```python
from build123d import *

# Parameters (mm, degrees)
DODANIE_WYCI_GNI_CIE1_DEPTH = 10
SZKIC2_R                    = 1.75
WYTNIJ_WYCI_GNI_CIE1_DEPTH  = 10


with BuildPart() as part:
    # Szkic1 → Dodanie-wyciągnięcie1 (new body)
    with BuildSketch(Plane(origin=(0, 0, 0), x_dir=(1, 0, 0), z_dir=(0, 1, 0))):
        with BuildLine():
            Line((22, -25), (-22, -25))
            ThreePointArc((-22, -25), (-24.121320344, -24.121320344), (-25, -22))
            Line((-25, -22), (-25, 22))
            ThreePointArc((-25, 22), (-24.121320344, 24.121320344), (-22, 25))
            Line((-22, 25), (22, 25))
            ThreePointArc((22, 25), (24.121320344, 24.121320344), (25, 22))
            Line((25, 22), (25, -22))
            ThreePointArc((25, -22), (24.121320344, -24.121320344), (22, -25))
        make_face()
    extrude(amount=DODANIE_WYCI_GNI_CIE1_DEPTH)

    # Szkic2 → Wytnij-wyciągnięcie1 (cut)
    with BuildSketch(Plane(origin=(0, 10, 0), x_dir=(1, 0, 0), z_dir=(0, 1, 0))):
        with Locations(Location((-20, 20, 0), (0, 0, 270))):
            Circle(SZKIC2_R)
        with Locations(Location((20, 20, 0), (0, 0, 270))):
            Circle(SZKIC2_R)
        with Locations(Location((20, -20, 0), (0, 0, 270))):
            Circle(SZKIC2_R)
        with Locations(Location((-20, -20, 0), (0, 0, 270))):
            Circle(SZKIC2_R)
        with BuildLine():
            Line((19.949804326, -0.416088747), (8.887895851, -0.416088747))
            ThreePointArc((8.887895851, -0.416088747), (8.238797705, -0.655384076), (7.900351868, -1.258745553))
            ThreePointArc((7.900351868, -1.258745553), (4.101739563, -6.868459256), (-2.638482905, -7.552377636))
            ThreePointArc((-2.638482905, -7.552377636), (-3.348489276, -7.571518902), (-3.866696101, -8.057252494))
            Line((-3.866696101, -8.057252494), (-8.71289149, -17.970981564))
            ThreePointArc((-8.71289149, -17.970981564), (-8.751315605, -18.759947091), (-8.20521309, -19.330661607))
            ThreePointArc((-8.20521309, -19.330661607), (10.963128103, -17.911164736), (20.947294543, -1.486893185))
            ThreePointArc((20.947294543, -1.486893185), (20.681516168, -0.734474647), (19.949804326, -0.416088747))
        make_face()
        with BuildLine():
            Line((19.918829975, 1.449846448), (8.910113622, 0.686816973))
            ThreePointArc((8.910113622, 0.686816973), (8.230490402, 0.892390127), (7.858638328, 1.497265385))
            ThreePointArc((7.858638328, 1.497265385), (3.997324324, 6.929747344), (-2.638482905, 7.552377636))
            ThreePointArc((-2.638482905, 7.552377636), (-3.348489276, 7.571518902), (-3.866696101, 8.057252494))
            Line((-3.866696101, 8.057252494), (-8.71289149, 17.970981564))
            ThreePointArc((-8.71289149, 17.970981564), (-8.751315605, 18.759947091), (-8.20521309, 19.330661607))
            ThreePointArc((-8.20521309, 19.330661607), (10.495454585, 18.189157019), (20.842168696, 2.569825685))
            ThreePointArc((20.842168696, 2.569825685), (20.621275551, 1.81133417), (19.918829975, 1.449846448))
        make_face()
        with BuildLine():
            Line((-11.206880821, -16.531076152), (-5.044437294, -7.377283299))
            ThreePointArc((-5.044437294, -7.377283299), (-4.882883076, -6.685636228), (-5.221309439, -6.061182041))
            ThreePointArc((-5.221309439, -6.061182041), (-8, 0), (-5.221309439, 6.061182041))
            ThreePointArc((-5.221309439, 6.061182041), (-4.882883076, 6.685636228), (-5.044437294, 7.377283299))
            Line((-5.044437294, 7.377283299), (-11.206880821, 16.531076152))
            ThreePointArc((-11.206880821, 16.531076152), (-11.870932952, 16.958835176), (-12.638237478, 16.771253783))
            ThreePointArc((-12.638237478, 16.771253783), (-21, 0), (-12.638237478, -16.771253783))
            ThreePointArc((-12.638237478, -16.771253783), (-11.870932952, -16.958835176), (-11.206880821, -16.531076152))
        make_face()
    extrude(amount=-WYTNIJ_WYCI_GNI_CIE1_DEPTH, mode=Mode.SUBTRACT)


solid = part.part
```
Can you work these out from the model? Positions are in its coordinate system, mm. A direction names the side the tool comes from. Coordinates: 2 decimals unless noted, no trailing zeros. Loops run counter-clockwise (first coordinate to the right, second up) from the corner with the lowest first, then second, coordinate; pieces in that order, holes last.
1) Thinking about a two-plate mould opening in X: for faces 3 (the flat face through (0, 0, 0)), 4 (the cylindrical face through (24.14, 4.93, 24.1)), 5 (the flat face through (-6.256, 5.07, 12.945)), which applies, pulls with the +X half, pulls with the -X half, needs draft (parallel to the pull), parting line crosses it, or undercut?
2) Imagine slicing it at C-C on x = -1. List the corners of the cut face in (y, z) for me.
3) Imagine slicing it at D-D on x = -6. List the corners of the cut face in (y, z) for me, plus the area to 3 significant figures.
4) Imagine slicing it at B-B on z = -20. List the corners of the cut face in (x, y) for me, plus the area to 3 significant figures.
5) Which directions (+Z, -Z, +X, -X, +Y, -Y) give clear straight access to the entire face, cutting with the end or side of a thin tool? Please do faces 1 (the flat face through (0, 5, -25)), 2 (the flat face through (-8.083, 5.07, -11.89)).
6) Imagine slicing it at A-A on x = -20. List the corners of the cut face in (y, z) for me, plus the area to 3 significant figures.
7) I need wall thicknesses on probe 1 along Z at (x, y) = (-19, 7.5); probe 2 along Z at (x, y) = (13, 3.5); probe 3 along X at (y, z) = (8.25, 9). Which ranges of each line are inside material? Lowest first, please.
Completed:
1. face 3: needs draft
1. face 4: pulls with the +X half
1. face 5: undercut
2. outline: (0, -25) - (10, -25) - (10, -20.98) - (0, -20.98) - close; (0, -7.94) - (10, -7.94) - (10, 7.94) - (0, 7.94) - close; (0, 20.98) - (10, 20.98) - (10, 25) - (0, 25) - close
3. outline: (0, -25) - (10, -25) - (10, -20.12) - (0, -20.12) - close; (0, -12.42) - (10, -12.42) - (10, -8.8) - (0, -8.8) - close; (0, -5.29) - (10, -5.29) - (10, 5.29) - (0, 5.29) - close; (0, 8.8) - (10, 8.8) - (10, 12.42) - (0, 12.42) - close; (0, 20.12) - (10, 20.12) - (10, 25) - (0, 25) - close
3. area: 276 mm2
4. outline: (-25, 0) - (-21.75, 0) - (-21.75, 10) - (-25, 10) - close; (-18.25, 0) - (-6.4, 0) - (-6.4, 10) - (-18.25, 10) - close; (6.4, 0) - (18.25, 0) - (18.25, 10) - (6.4, 10) - close; (21.75, 0) - (25, 0) - (25, 10) - (21.75, 10) - close
4. area: 302 mm2
5. face 1: -Z, +X, -X, +Y, -Y
5. face 2: +Y, -Y
6. outline: (0, -25) - (10, -25) - (10, -21.75) - (0, -21.75) - close; (0, -18.25) - (10, -18.25) - (10, -6.4) - (0, -6.4) - close; (0, 6.4) - (10, 6.4) - (10, 18.25) - (0, 18.25) - close; (0, 21.75) - (10, 21.75) - (10, 25) - (0, 25) - close
6. area: 302 mm2
7. probe 1: z = -25 to -21.44, -18.56 to -8.94, 8.94 to 18.56, 21.44 to 25
7. probe 2: z = -25 to -16.49, -0.97 to 0.42, 16.49 to 25
7. probe 3: x = -25 to -18.97, -6.14 to -4.33, 18.97 to 25
